Source: CAD feature listing. Evaluate the final solid. Frame: model axes, mm. A direction names the side the tool comes from. Coordinates: 2 decimals unless noted, no trailing zeros. Order: outer loops, then holes, each group sorted by start corner. A loop starts at its lowest first (then second) coordinate and runs counter-clockwise, first axis right, second up.
Item 1: Contact query for flat-ended pins moving along their axis: P1, Ø2, axis at y = 2.5, z = -41, coming from the +X side; P2, Ø1, axis at x = -18, y = 5, coming from the -Z side; P3, Ø3, axis at x = -29, y = 4, coming from the +Z side. Output: stop coordinate, or through.
Item 2: Section C-C on x = 18. Return the cut outline in (y, z), then the cut area to 3 significant figures.
Item 3: Ray query, line 1 (Z direction, x = -19, y = 1.25); line 2 (X direction, y = 2.8, z = 24); line 3 (X direction, y = 1.5, z = -19). Return the intervals inside material, ascending.
Item 4: Reachability of faces 1 (the flat face through (2, 5, 50)), 2 (the flat face through (0, 2, -12.5)), 3 (the flat face through (-8, 2, 7)) from +Z, -Z, +X, -X, +Y, -Y: full face, straight path, thin tool, end or side. Return the list, or none.
Item 5: Section A-A on z = 0. Return the cut outline in (x, y).
Item 6: Section D-D on z = 18. Return the cut outline in (x, y).
Item 7: Section B-B on x = -18. Return the cut outline in (y, z), then the cut area to 3 significant figures.
from build123d import *

# Parameters (mm, degrees)
SKETCH1_R                       = 54
BASE_PLATE_DEPTH                = 8
HOLE_PATTERN_R                  = 2
MOTOR_MOUNT_HOLES_DEPTH         = 77.785415282
SKETCH3_R                       = 1.375
SKETCH3_R_2                     = 4
ENCODER_MOUNTING_HOLES_DEPTH    = 77.785415282
SKETCH4_W                       = 22
SKETCH4_H                       = 8
ENCODER_WIRE_PASS_THROUGH_DEPTH = 5
MOTOR_WIRE_PASS_THROUGH_DEPTH   = 77.785415282
SKETCH6_W                       = 11.998985868
SKETCH6_H                       = 14
CUT_EXTRUDE6_DEPTH              = 2
CUT_EXTRUDE7_DEPTH              = 2
CUT_EXTRUDE8_DEPTH              = 3
SKETCH10_W                      = 23
SKETCH10_H                      = 29
CUT_EXTRUDE9_DEPTH              = 3


with BuildPart() as part:
    # Sketch1 → Base Plate (new body)
    with BuildSketch(Plane(origin=(0, 0, 0), x_dir=(1, 0, 0), z_dir=(0, 1, 0))):
        with Locations(Location((0, 0, 0), (0, 0, 270))):
            Circle(SKETCH1_R)
    extrude(amount=BASE_PLATE_DEPTH)

    # Hole Pattern → Motor Mount Holes (cut, through all)
    with BuildSketch(Plane.XZ):
        with Locations(Location((0, 48, 0), (0, 0, 270))):
            Circle(HOLE_PATTERN_R)
        with Locations(Location((41.569219382, 24, 0), (0, 0, 270))):
            Circle(HOLE_PATTERN_R)
        with Locations(Location((41.569219382, -24, 0), (0, 0, 270))):
            Circle(HOLE_PATTERN_R)
        with Locations(Location((0, -48, 0), (0, 0, 270))):
            Circle(HOLE_PATTERN_R)
        with Locations(Location((-41.569219382, -24, 0), (0, 0, 270))):
            Circle(HOLE_PATTERN_R)
        with Locations(Location((-41.569219382, 24, 0), (0, 0, 270))):
            Circle(HOLE_PATTERN_R)
        with Locations(Location((0, 18, 0), (0, 0, 270))):
            Circle(HOLE_PATTERN_R)
        with Locations(Location((18, 0, 0), (0, 0, 270))):
            Circle(HOLE_PATTERN_R)
        with Locations(Location((-18, 0, 0), (0, 0, 270))):
            Circle(HOLE_PATTERN_R)
    extrude(amount=-MOTOR_MOUNT_HOLES_DEPTH, mode=Mode.SUBTRACT)

    # Sketch3 → Encoder mounting holes (cut, through all)
    with BuildSketch(Plane(origin=(0, 8, 0), x_dir=(1, 0, 0), z_dir=(0, 1, 0))):
        with Locations(Location((-9, 5.5, 0), (0, 0, 270))):
            Circle(SKETCH3_R)
        with Locations(Location((9, 5.5, 0), (0, 0, 270))):
            Circle(SKETCH3_R)
        with Locations(Location((9, -5.5, 0), (0, 0, 270))):
            Circle(SKETCH3_R)
        with Locations(Location((-9, -5.5, 0), (0, 0, 270))):
            Circle(SKETCH3_R)
        with Locations(Location((0, 0, 0), (0, 0, 270))):
            Circle(SKETCH3_R_2)
    extrude(amount=-ENCODER_MOUNTING_HOLES_DEPTH, mode=Mode.SUBTRACT)

    # Sketch4 → Encoder Wire Pass through (cut)
    with BuildSketch(Plane(origin=(0, 0, 0), x_dir=(1, 0, 0), z_dir=(0, 1, 0))):
        with Locations((0, 16.5)):
            Rectangle(SKETCH4_W, SKETCH4_H)
    extrude(amount=ENCODER_WIRE_PASS_THROUGH_DEPTH, mode=Mode.SUBTRACT)

    # Sketch5 → Motor Wire pass through (cut, through all)
    with BuildSketch(Plane(origin=(0, 8, 0), x_dir=(1, 0, 0), z_dir=(0, 1, 0))):
        Polygon((-33.587572106, 20.152543264), (-28.637824638, 15.202795796), (-15.202795796, 28.637824638), (-20.152543264, 33.587572106), align=None)
    extrude(amount=-MOTOR_WIRE_PASS_THROUGH_DEPTH, mode=Mode.SUBTRACT)

    # Sketch6 → Cut-Extrude6 (cut)
    with BuildSketch(Plane(origin=(0, 8, 0), x_dir=(1, 0, 0), z_dir=(0, 1, 0))):
        with Locations((0, 12.5)):
            Rectangle(SKETCH6_W, SKETCH6_H)
    extrude(amount=-CUT_EXTRUDE6_DEPTH, mode=Mode.SUBTRACT)

    # Sketch7 → Cut-Extrude7 (cut)
    with BuildSketch(Plane.XZ):
        Polygon((7.556624327, 3), (10.443375673, 3), (11.886751346, 5.5), (10.443375673, 8), (7.556624327, 8), (6.113248654, 5.5), align=None)
        Polygon((10.443375673, -8), (11.886751346, -5.5), (10.443375673, -3), (7.556624327, -3), (6.113248654, -5.5), (7.556624327, -8), align=None)
        Polygon((-7.556624327, -8), (-6.113248654, -5.5), (-7.556624327, -3), (-10.443375673, -3), (-11.886751346, -5.5), (-10.443375673, -8), align=None)
        Polygon((-7.556624327, 3), (-6.113248654, 5.5), (-7.556624327, 8), (-10.443375673, 8), (-11.886751346, 5.5), (-10.443375673, 3), align=None)
    extrude(amount=-CUT_EXTRUDE7_DEPTH, mode=Mode.SUBTRACT)

    # Sketch9 → Cut-Extrude8 (cut)
    with BuildSketch(Plane.XZ.offset(-8)):
        Polygon((39.548493439, -27.5), (43.589945324, -27.5), (45.610671266, -24), (43.589945324, -20.5), (39.548493439, -20.5), (37.527767497, -24), align=None)
        Polygon((-4.041451884, -48), (-2.020725942, -51.5), (2.020725942, -51.5), (4.041451884, -48), (2.020725942, -44.5), (-2.020725942, -44.5), align=None)
        Polygon((43.589945324, 20.5), (45.610671266, 24), (43.589945324, 27.5), (39.548493439, 27.5), (37.527767497, 24), (39.548493439, 20.5), align=None)
        Polygon((4.041451884, 48), (2.020725942, 51.5), (-2.020725942, 51.5), (-4.041451884, 48), (-2.020725942, 44.5), (2.020725942, 44.5), align=None)
        Polygon((-39.548493439, 27.5), (-43.589945324, 27.5), (-45.610671266, 24), (-43.589945324, 20.5), (-39.548493439, 20.5), (-37.527767497, 24), align=None)
        Polygon((-43.589945324, -20.5), (-45.610671266, -24), (-43.589945324, -27.5), (-39.548493439, -27.5), (-37.527767497, -24), (-39.548493439, -20.5), align=None)
    extrude(amount=CUT_EXTRUDE8_DEPTH, mode=Mode.SUBTRACT)

    # Sketch10 → Cut-Extrude9 (cut)
    with BuildSketch(Plane(origin=(0, 8, 0), x_dir=(1, 0, 0), z_dir=(0, 1, 0))):
        with Locations((0, 6.5)):
            Rectangle(SKETCH10_W, SKETCH10_H)
    extrude(amount=-CUT_EXTRUDE9_DEPTH, mode=Mode.SUBTRACT)


solid = part.part
Answer list:
1. P1: stops at x = 36.28
1. P2: stops at z = -51.09
1. P3: stops at z = 46.47
2. outline: (0, -50.91) - (8, -50.91) - (8, -2) - (0, -2) - close; (0, 2) - (8, 2) - (8, 50.91) - (0, 50.91) - close
2. area: 783 mm2
3. line 1: z = -50.55 to -32.44, -24.84 to -1.73, 1.73 to 50.55
3. line 2: x = -48.37 to -43.57, -39.57 to 39.57, 43.57 to 48.37
3. line 3: x = -50.55 to -32.44, -24.84 to -11, 11 to 50.55
4. face 1: +Y
4. face 2: +Y, -Y
4. face 3: -Y
5. outline: (-54, 0) - (-20, 0) - (-20, 8) - (-54, 8) - close; (-16, 0) - (-4, 0) - (-4, 5) - (-11.5, 5) - (-11.5, 8) - (-16, 8) - close; (4, 0) - (16, 0) - (16, 8) - (11.5, 8) - (11.5, 5) - (4, 5) - close; (20, 0) - (54, 0) - (54, 8) - (20, 8) - close
6. outline: (-50.91, 0) - (-2, 0) - (-2, 8) - (-50.91, 8) - close; (2, 0) - (50.91, 0) - (50.91, 8) - (2, 8) - close
7. outline: (0, -50.91) - (8, -50.91) - (8, -31.44) - (0, -31.44) - close; (0, -25.84) - (8, -25.84) - (8, -2) - (0, -2) - close; (0, 2) - (8, 2) - (8, 50.91) - (0, 50.91) - close
7. area: 738 mm2
